Autodesk Fusion 360 part; units mm, degrees
sketch "Sketch1" plane through (0, 0, 0) normal (0, 0, 1) x (1, 0, 0)
  line L0 (140, 280) -> (-140, 280)
  line L1 (-140, 280) -> (-140, -280)
  line L2 (-140, -280) -> (140, -280)
  line L3 (140, -280) -> (140, 280)
  line L4 (140, 280) -> (-140, -280) construction
  line L5 (-140, 280) -> (140, -280) construction
  dimension "d1" = 140
  dimension "d2" = 280
extrude "Extrude1" add sketch "Sketch1" along normal blind 20
fillet "Fillet1" radius 40 4 edges at (140, -280, 10) (-140, -280, 10) (140, 280, 10) (-140, 280, 10)
sketch "Sketch2" plane through (0, -280, 0) normal (0, -1, 0) x (1, 0, 0)
  line L0 (-100, 20) -> (-100, 0)
  line L1 (-100, 0) -> (100, 0)
  line L2 (100, 0) -> (100, 20)
  line L3 (100, 20) -> (-100, 20)
  line L4 (10, 15) -> (-10, 15)
  line L5 (-10, 5) -> (10, 5)
  line L6 (10, 15) -> (-10, 5) construction
  line L7 (-10, 15) -> (10, 5) construction
  arc A0 (10, 5) -> (10, 15) centre (8.875, 10) ccw
  line L8 (0, 15) -> (0, 5) construction
  arc A1 (-10, 15) -> (-10, 5) centre (-8.875, 10) ccw
  circle A2 centre (-30, 10) radius 3.8849
  circle A3 centre (-42.5, 10) radius 3.8849
  circle A4 centre (-55, 10) radius 3.8849
  circle A5 centre (30, 10) radius 3.8849
  circle A6 centre (42.5, 10) radius 3.8849
  circle A7 centre (55, 10) radius 3.8849
  circle A8 centre (67.5, 10) radius 3.8849
  circle A9 centre (80, 10) radius 3.8849
  point P0 (0, 10)
  dimension "d7" = 20
  dimension "d8" = 5.125
  dimension "d9" = 10
  dimension "d10" = 5
  dimension "d11" = 100
  dimension "d12" = 10
  dimension "d17" = -25
  dimension "d18" = 0
  dimension "d21" = 50
  dimension "d22" = 0
extrude "Extrude2" cut sketch "Sketch2" against normal blind 13 contours L4 L5 A0 A1
extrude "Extrude3" cut sketch "Sketch2" against normal blind 2 contours A2 | A3 | A4 | A5 | A6 | A7 | A8 | A9
sketch "Sketch3" plane through (140, 0, 0) normal (1, 0, 0) x (0, 1, 0)
  line L0 (240, 0) -> (240, 20)
  line L1 (240, 20) -> (-240, 20)
  line L2 (-240, 20) -> (-240, 0)
  line L3 (-240, 0) -> (240, 0)
  line L4 (-150, 4.2611) -> (-100, 4.2611)
  arc A0 (-100, 4.2611) -> (-100, 15.7389) centre (-100, 10) ccw
  line L5 (-100, 15.7389) -> (-150, 15.7389)
  arc A1 (-150, 15.7389) -> (-150, 4.2611) centre (-150, 10) ccw
  line L6 (-150, 10) -> (-100, 10) construction
  line L7 (50, 4.2841) -> (110, 4.2841)
  arc A2 (110, 4.2841) -> (110, 15.7159) centre (110, 10) ccw
  line L8 (110, 15.7159) -> (50, 15.7159)
  arc A3 (50, 15.7159) -> (50, 4.2841) centre (50, 10) ccw
  line L9 (50, 10) -> (110, 10) construction
  dimension "d27" = 11.4319
extrude "Extrude4" cut sketch "Sketch3" against normal blind 1 contours L4 A0 L5 A1
extrude "Extrude5" add sketch "Sketch3" along normal blind 5 contours L7 A2 L8 A3
sketch "Sketch4" plane through (-140, 0, 0) normal (-1, 0, 0) x (0, -1, 0)
  line L0 (-240, 20) -> (-240, 0)
  line L1 (-240, 0) -> (240, 0)
  line L2 (240, 0) -> (240, 20)
  line L3 (240, 20) -> (-240, 20)
  line L4 (-130, 4.0036) -> (-90, 4.0036)
  arc A0 (-90, 4.0036) -> (-90, 15.9964) centre (-90, 10) ccw
  line L5 (-90, 15.9964) -> (-130, 15.9964)
  arc A1 (-130, 15.9964) -> (-130, 4.0036) centre (-130, 10) ccw
  line L6 (-130, 10) -> (-90, 10) construction
  line L7 (-77.5677, 20) -> (-77.5677, 0) construction
  arc A2 (-65.1354, 15.9964) -> (-65.1354, 4.0036) centre (-65.1354, 10) ccw
  line L8 (-65.1354, 15.9964) -> (-25.1354, 15.9964)
  arc A3 (-25.1354, 4.0036) -> (-25.1354, 15.9964) centre (-25.1354, 10) ccw
  line L9 (-25.1354, 4.0036) -> (-65.1354, 4.0036)
  line L10 (-177, 4.5) -> (-170, 4.5)
  arc A4 (-170, 4.5) -> (-170, 15.5) centre (-170, 10) ccw
  line L11 (-170, 15.5) -> (-177, 15.5)
  arc A5 (-177, 15.5) -> (-177, 4.5) centre (-177, 10) ccw
  line L12 (-177, 10) -> (-170, 10) construction
  dimension "d30" = 40
  dimension "d31" = 11
extrude "Extrude6" add sketch "Sketch4" along normal blind 4 contours L4 A0 L5 A1 | A2 L8 A3 L9 | L10 A4 L11 A5
sketch "Sketch5" plane through (0, 0, 0) normal (0, 0, -1) x (1, 0, 0)
  arc A0 (-140, -240) -> (-100, -280) centre (-100, -240) ccw
  line L0 (-100, -280) -> (100, -280)
  arc A1 (100, -280) -> (140, -240) centre (100, -240) ccw
  line L1 (140, -240) -> (140, 240)
  arc A2 (140, 240) -> (100, 280) centre (100, 240) ccw
  line L2 (100, 280) -> (-100, 280)
  arc A3 (-100, 280) -> (-140, 240) centre (-100, 240) ccw
  line L3 (-140, 240) -> (-140, -240)
  line L4 (126.7816, -230) -> (126.7816, -165)
  arc A4 (126.7816, -165) -> (56.6683, -165) centre (91.725, -165) ccw
  line L5 (56.6683, -165) -> (56.6683, -230)
  arc A5 (56.6683, -230) -> (126.7816, -230) centre (91.725, -230) ccw
  line L6 (91.725, -230) -> (91.725, -165) construction
  dimension "d34" = 35.0567
  dimension "d36" = 75
  dimension "d38" = 50
extrude "Extrude7" add sketch "Sketch5" along normal blind 5 contours L4 A4 L5 A5
sketch "Sketch6" plane through (0, 0, -5) normal (0, 0, -1) x (1, 0, 0)
  arc A0 (56.6683, -230) -> (126.7816, -230) centre (91.725, -230) ccw
  line L0 (126.7816, -230) -> (126.7816, -165)
  arc A1 (126.7816, -165) -> (56.6683, -165) centre (91.725, -165) ccw
  line L1 (56.6683, -165) -> (56.6683, -230)
  circle A2 centre (91.725, -230) radius 28.5736
  line L2 (91.725, -197.5847) -> (60, -197.5847) construction
  circle A3 centre (91.725, -165.1693) radius 28.5736
extrude "Extrude8" add sketch "Sketch6" along normal blind 5 contours A2 | A3
sketch "Sketch7" plane through (0, 0, 0) normal (0, 0, -1) x (1, 0, 0)
  line L0 (56.6683, -230) -> (56.6683, -165)
  arc A0 (126.7816, -165) -> (56.6683, -165) centre (91.725, -165) ccw
  line L1 (126.7816, -165) -> (126.7816, -230)
  arc A1 (56.6683, -230) -> (126.7816, -230) centre (91.725, -230) ccw
  arc A2 (-140, -240) -> (-100, -280) centre (-100, -240) ccw
  line L2 (-100, -280) -> (100, -280)
  arc A3 (100, -280) -> (140, -240) centre (100, -240) ccw
  line L3 (140, -240) -> (140, 240)
  arc A4 (140, 240) -> (100, 280) centre (100, 240) ccw
  line L4 (100, 280) -> (-100, 280)
  arc A5 (-100, 280) -> (-140, 240) centre (-100, 240) ccw
  line L5 (-140, 240) -> (-140, -240)
  circle A6 centre (35.4902, -197.5) radius 7.4639
extrude "Extrude9" add sketch "Sketch7" along normal blind 1.5 contours A6
sketch "Sketch8" plane through (0, 0, 20) normal (0, 0, 1) x (-1, 0, 0)
  arc A0 (100, -280) -> (140, -240) centre (100, -240) ccw
  line L0 (140, -240) -> (140, 240)
  arc A1 (140, 240) -> (100, 280) centre (100, 240) ccw
  line L1 (100, 280) -> (-100, 280)
  arc A2 (-100, 280) -> (-140, 240) centre (-100, 240) ccw
  line L2 (-140, 240) -> (-140, -240)
  arc A3 (-140, -240) -> (-100, -280) centre (-100, -240) ccw
  line L3 (-100, -280) -> (100, -280)
  line L4 (25, -258.4273) -> (-25, -258.4273)
  arc A4 (-25, -258.4273) -> (-25, -271.5727) centre (-25, -265) ccw
  line L5 (-25, -271.5727) -> (25, -271.5727)
  arc A5 (25, -271.5727) -> (25, -258.4273) centre (25, -265) ccw
  line L6 (25, -265) -> (-25, -265) construction
extrude "Extrude10" add sketch "Sketch8" along normal blind 1 contours L4 A4 L5 A5
sketch "Sketch9" plane through (0, 0, 0) normal (0, 0, -1) x (1, 0, 0)
  circle A0 centre (35.4902, -197.5) radius 7.4639
  line L0 (56.6683, -230) -> (56.6683, -165)
  arc A1 (126.7816, -165) -> (56.6683, -165) centre (91.725, -165) ccw
  line L1 (126.7816, -165) -> (126.7816, -230)
  arc A2 (56.6683, -230) -> (126.7816, -230) centre (91.725, -230) ccw
  arc A3 (-140, -240) -> (-100, -280) centre (-100, -240) ccw
  line L2 (-100, -280) -> (100, -280)
  arc A4 (100, -280) -> (140, -240) centre (100, -240) ccw
  line L3 (140, -240) -> (140, 240)
  arc A5 (140, 240) -> (100, 280) centre (100, 240) ccw
  line L4 (100, 280) -> (-100, 280)
  arc A6 (-100, 280) -> (-140, 240) centre (-100, 240) ccw
  line L5 (-140, 240) -> (-140, -240)
  spline S0 degree 3 poles (-24.7768, 20.7597) (-21.4828, 25.6809) (-17.9903, 30.4831) (-12.6722, 30.5625) knots 0 0 0 0 1 1 1 1
  spline S1 degree 3 poles (-12.6722, 30.5625) (-7.354, 30.6815) (-5.6475, 27.4272) (0.385, 27.4272) knots 0 0 0 0 1 1 1 1
  spline S2 degree 3 poles (0.385, 27.4272) (6.4572, 27.4272) (8.3225, 30.4831) (13.363, 30.6815) knots 0 0 0 0 1 1 1 1
  spline S3 degree 3 poles (13.363, 30.6815) (18.562, 30.88) (22.4911, 25.4428) (25.8248, 20.6406) knots 0 0 0 0 1 1 1 1
  spline S4 degree 3 poles (25.8248, 20.6406) (32.6114, 10.8378) (37.8105, -7.22) (30.8255, -19.3644) knots 0 0 0 0 1 1 1 1
  spline S5 degree 3 poles (30.8255, -19.3644) (27.3726, -25.3969) (21.1814, -29.2069) (14.4742, -29.326) knots 0 0 0 0 1 1 1 1
  spline S6 degree 3 poles (14.4742, -29.326) (9.3941, -29.4053) (4.5522, -25.8731) (1.4169, -25.8731) knots 0 0 0 0 1 1 1 1
  spline S7 degree 3 poles (1.4169, -25.8731) (-1.6787, -25.8731) (-7.5525, -30.1197) (-13.704, -29.4847) knots 0 0 0 0 1 1 1 1
  spline S8 degree 3 poles (-13.704, -29.4847) (-16.2837, -29.3657) (-23.5068, -28.4528) (-28.1503, -21.6266) knots 0 0 0 0 1 1 1 1
  spline S9 degree 3 poles (-28.1503, -21.6266) (-27.7931, -21.3885) (-19.5381, -16.5466) (-19.6175, -6.5056) knots 0 0 0 0 1 1 1 1
  spline S10 degree 3 poles (-19.6175, -6.5056) (-19.7365, 5.48) (-30.1347, 9.4884) (-30.2537, 9.5281) knots 0 0 0 0 1 1 1 1
  spline S11 degree 3 poles (-30.2537, 9.5281) (-30.1347, 9.8059) (-28.5868, 15.2431) (-24.7768, 20.7597) knots 0 0 0 0 1 1 1 1
  spline S12 degree 3 poles (-2.1153, -42.7403) (-5.0125, -46.0344) (-9.8147, -48.5347) (-13.7834, -48.6935) knots 0 0 0 0 1 1 1 1
  spline S13 degree 3 poles (-13.7834, -48.6935) (-14.2993, -44.05) (-12.434, -39.3669) (-9.6559, -36.0331) knots 0 0 0 0 1 1 1 1
  spline S14 degree 3 poles (-9.6559, -36.0331) (-6.9175, -32.6597) (-2.3931, -30.0403) (2.0519, -30.3975) knots 0 0 0 0 1 1 1 1
  spline S15 degree 3 poles (2.0519, -30.3975) (2.6472, -34.9616) (0.4247, -39.7241) (-2.1153, -42.7403) knots 0 0 0 0 1 1 1 1
For this review, take the finished solid that the model builds, in its own axes (mm). A direction names the side the tool comes from. Coordinates: 2 decimals unless noted, no trailing zeros. Write each loop counter-clockwise with the first axis right and the second up, starting at its lowest first coordinate (ties: lowest second). Pieces come first, ordered by that corner, then holes. Notation, with made-up numbers: (1.5, -26.75) -> (41.5, -26.75) arc R20 cw to (41.5, -9.75) -> close; hole circle Ø6 at (81, -38.5). An arc over 180 degrees is marked (long way). Put each result on its own line as item: value.
Q1. Take a section at B-B, the plane x = -92.5. State the section outline as (y, z) points.
From the geometry:
outline: (-280, 0) -> (280, 0) -> (280, 20) -> (-280, 20) -> close
Q2. Tool access review of faces 5 (the cylindrical face through (92.5, 265.05, -2.46)), 6 (the cylindrical face through (104.91, 204.65, -7.46)), 7 (the flat face through (139, -125, 10)), 8 (the flat face through (0, -267, 10)), 9 (the flat face through (35, 197, -1.5)): name each direction out of +Z, -Z, +X, -X, +Y, -Y from which nothing blocks a thin tool from reaching the whole face with its end or side.
From the geometry:
face 5: -Z, +Y
face 6: -Z
face 7: +X
face 8: -Y
face 9: -Z, -X, +Y, -Y
Q3. Take a section at C-C, the plane y = -172.5. State the section outline as (x, z) points.
From the geometry:
outline: (-140, 0) -> (140, 0) -> (140, 20) -> (-140, 20) -> close
Q4. Take a section at A-A, the plane y = -108. State the section outline as (x, z) points.
From the geometry:
outline: (-140, 0) -> (140, 0) -> (140, 4.26) -> (139, 4.26) -> (139, 15.74) -> (140, 15.74) -> (140, 20) -> (-140, 20) -> close
Q5. The part is to be moulded in two halves that separate along Z. For faces 1 (the cylindrical face through (14, -274, 10)), 2 (the flat face through (91, 197, -5)), 3 (the flat face through (0, -274, 15)), 4 (the flat face through (-140, 3, 10)), say which applies: +Z half, -Z half, draft (parallel to the pull), parting line (faces both ways), or undercut.
From the geometry:
face 1: undercut
face 2: -Z half
face 3: undercut
face 4: draft
Q6. Wall thickness on L1, parallel to Z at x = 30, y = -279; L2, parallel to Z at x = -29, y = -41.5; L3, parallel to X at y = -114.5, z = 12: over which ranges is each line inside the solid? List them lowest first.
From the geometry:
L1: z = 0 to 6.12, 13.88 to 20
L2: z = 0 to 20
L3: x = -140 to 139
Q7. Clearance check with flat-ended pins moving along their axes: pin 1 Ø6.5 at (x, y) = (-3, -275) entering from +Z; pin 2 Ø8 at (x, z) = (3, 8.5) entering from -Y; pin 3 Ø1.5 at (x, y) = (-11, -152.5) entering from -Z; pin 4 Ø5 at (x, z) = (104.5, 11.5) entering from +Y. State where each tip first meets the part, or that it passes through.
From the geometry:
pin 1: stops at z = 20
pin 2: stops at y = -280
pin 3: stops at z = 0
pin 4: stops at y = 279.95
